```python
from build123d import *

# Parameters (mm, degrees)
SKETCH1_R           = 5.1
BOSS_EXTRUDE1_DEPTH = 5
CUT_EXTRUDE1_START  = -2.3
SKETCH2_R           = 7.5
CUT_EXTRUDE1_DEPTH  = 33.942020373
BOSS_EXTRUDE2_DEPTH = 12
SKETCH4_R           = 5
SKETCH4_R_2         = 1.75
SKETCH4_R_3         = 2.5
CUT_EXTRUDE2_DEPTH  = 37.455291152
FILLET1_R           = 1
SKETCH5_W           = 20
SKETCH5_H           = 6.532082626
CUT_EXTRUDE3_DEPTH  = 37.672994655
FILLET2_R           = 2
FILLET3_R           = 6


with BuildPart() as part:
    # Sketch1 → Boss-Extrude1 (new body)
    with BuildSketch(Plane.XY):
        with BuildLine():
            Line((-27, -16), (27, -16))
            ThreePointArc((27, -16), (29.828427125, -14.828427125), (31, -12))
            Line((31, -12), (31, 12))
            ThreePointArc((31, 12), (29.828427125, 14.828427125), (27, 16))
            Line((27, 16), (-27, 16))
            ThreePointArc((-27, 16), (-29.828427125, 14.828427125), (-31, 12))
            Line((-31, 12), (-31, -12))
            ThreePointArc((-31, -12), (-29.828427125, -14.828427125), (-27, -16))
        make_face()
        with Locations((-20, 9)):
            Circle(SKETCH1_R, mode=Mode.SUBTRACT)
        with Locations((20, -9)):
            Circle(SKETCH1_R, mode=Mode.SUBTRACT)
        with Locations((-20, -9)):
            Circle(SKETCH1_R, mode=Mode.SUBTRACT)
        with Locations((20, 9)):
            Circle(SKETCH1_R, mode=Mode.SUBTRACT)
    extrude(amount=BOSS_EXTRUDE1_DEPTH)

    # Sketch2 → Cut-Extrude1 (cut, through all)
    with BuildSketch(Plane(origin=(0, 0, 0), x_dir=(-1, 0, 0), z_dir=(0, 0, -1)).offset(CUT_EXTRUDE1_START)):
        with Locations((20, 9)):
            Circle(SKETCH2_R)
        with Locations((-20, 9)):
            Circle(SKETCH2_R)
        with Locations((-20, -9)):
            Circle(SKETCH2_R)
        with Locations((20, -9)):
            Circle(SKETCH2_R)
    extrude(amount=-CUT_EXTRUDE1_DEPTH, mode=Mode.SUBTRACT)

    # Sketch3 → Boss-Extrude2 (add, symmetric)
    with BuildSketch(Plane(origin=(0, 0, 0), x_dir=(0, 0, -1), z_dir=(1, 0, 0))):
        Polygon((-5, 16), (-9.770224884, -8.540679586), (-5, -9.467917374), align=None)
        Polygon((0, 16), (-5, 16), (-4.427573014, 18.94488155), (0, 18.94488155), align=None)
    extrude(amount=BOSS_EXTRUDE2_DEPTH, both=True)

    # Sketch4 → Cut-Extrude2 (cut, through all)
    with BuildSketch(Plane(origin=(0, 1.519045647, 7.814812384), x_dir=(1, 0, 0), z_dir=(0, 0.19080899537654522, 0.981627183447664))):
        with Locations(Location((0, 4, 0), (0, 0, 270))):
            Circle(SKETCH4_R)
        with Locations(Location((0, 13, 0), (0, 0, 270))):
            Circle(SKETCH4_R_2)
        with Locations(Location((8, 4, 0), (0, 0, 270))):
            Circle(SKETCH4_R_2)
        with Locations(Location((0, -5, 0), (0, 0, 270))):
            Circle(SKETCH4_R_2)
        with Locations(Location((-8, 4, 0), (0, 0, 270))):
            Circle(SKETCH4_R_2)
        with Locations(Location((-6.686187475, -2.686187475, 0), (0, 0, 270))):
            Circle(SKETCH4_R_3)
        with Locations(Location((6.686187475, -2.686187475, 0), (0, 0, 90))):
            Circle(SKETCH4_R_3)
        with Locations(Location((6.686187475, 10.686187475, 0), (0, 0, 270))):
            Circle(SKETCH4_R_3)
        with Locations(Location((-6.686187475, 10.686187475, 0), (0, 0, 90))):
            Circle(SKETCH4_R_3)
    extrude(amount=-CUT_EXTRUDE2_DEPTH, mode=Mode.SUBTRACT)

    # Fillet1
    # the kernel refuses this fillet: 1 mm, written as the material it adds along each edge
    with BuildSketch(Plane(origin=(12, 16, 0), x_dir=(1, 0, 0), z_dir=(0, 0, 1))) as fillet1_piece_1_section:
        with BuildLine():
            CenterArc((FILLET1_R, FILLET1_R), FILLET1_R, 180, 90)
            Line((0, FILLET1_R), (0, 0))
            Line((0, 0), (FILLET1_R, 0))
        make_face()
    fillet1_piece_1 = extrude(amount=5, mode=Mode.PRIVATE)
    fillet1_piece_1 = split(fillet1_piece_1, bisect_by=Plane(origin=(12.227463764, 16.688764384, 4.866117766), z_dir=(0, -0.19080899537654517, -0.981627183447664)), keep=Keep.TOP, mode=Mode.PRIVATE)
    add(fillet1_piece_1)
    with BuildSketch(Plane(origin=(-12, 16, 0), x_dir=(-1, 0, 0), z_dir=(0, 0, 1))) as fillet1_piece_2_section:
        with BuildLine():
            CenterArc((FILLET1_R, -FILLET1_R), FILLET1_R, 90, 90)
            Line((0, -FILLET1_R), (0, 0))
            Line((0, 0), (FILLET1_R, 0))
        make_face()
    fillet1_piece_2 = extrude(amount=5, mode=Mode.PRIVATE)
    fillet1_piece_2 = split(fillet1_piece_2, bisect_by=Plane(origin=(-12.227463764, 16.688764384, 4.866117766), z_dir=(0, -0.19080899537654517, -0.981627183447664)), keep=Keep.TOP, mode=Mode.PRIVATE)
    add(fillet1_piece_2)
    # the kernel refuses this fillet: 1 mm, written as the material it takes off along each edge
    with BuildSketch(Plane(origin=(12, 18.94488155, 6.927573014), x_dir=(0, -1, 0), z_dir=(0, 0, -1))) as fillet1_2_piece_1:
        with BuildLine():
            CenterArc((FILLET1_R, FILLET1_R), FILLET1_R, 180, 90)
            Line((0, FILLET1_R), (0, 0))
            Line((0, 0), (FILLET1_R, 0))
        make_face()
    extrude(amount=9.427573014, mode=Mode.SUBTRACT)
    with BuildSketch(Plane(origin=(-12, 18.94488155, 6.927573014), x_dir=(0, -1, 0), z_dir=(0, 0, -1))) as fillet1_2_piece_2:
        with BuildLine():
            CenterArc((FILLET1_R, -FILLET1_R), FILLET1_R, 90, 90)
            Line((0, -FILLET1_R), (0, 0))
            Line((0, 0), (FILLET1_R, 0))
        make_face()
    extrude(amount=9.427573014, mode=Mode.SUBTRACT)

    # Sketch5 → Cut-Extrude3 (cut, through all)
    with BuildSketch(Plane.XY.offset(5)):
        with Locations((0, -12.733958687)):
            Rectangle(SKETCH5_W, SKETCH5_H)
    extrude(amount=-CUT_EXTRUDE3_DEPTH, mode=Mode.SUBTRACT)

    # Fillet2
    fillet2_edges = [part.edges().sort_by_distance(p)[0] for p in [
        (-10, -16, 2.5),
        (-10, -9.467917374, 2.5),
        (10, -9.467917374, 2.5),
        (10, -16, 2.5),
    ]]
    fillet(fillet2_edges, radius=FILLET2_R)

    # Fillet3
    # the kernel refuses this fillet: 6 mm, written as the material it takes off along each edge
    with BuildSketch(Plane(origin=(-12, -5.678544656, 24.494632636), x_dir=(1, 0, 0), z_dir=(0, -0.19080899537654505, -0.981627183447664))) as fillet3_piece_1_section:
        with BuildLine():
            CenterArc((FILLET3_R, -FILLET3_R), FILLET3_R, 90, 90)
            Line((0, -FILLET3_R), (0, 0))
            Line((0, 0), (FILLET3_R, 0))
        make_face()
    fillet3_piece_1 = extrude(amount=34.859507728, mode=Mode.PRIVATE)
    fillet3_piece_1 = split(fillet3_piece_1, bisect_by=Plane(origin=(-10.628321285, -7.717365946, 5), z_dir=(0, 0, 1)), keep=Keep.TOP, mode=Mode.PRIVATE)
    add(fillet3_piece_1, mode=Mode.SUBTRACT)
    with BuildSketch(Plane(origin=(12, -5.678544656, 24.494632636), x_dir=(-1, 0, 0), z_dir=(0, -0.19080899537654505, -0.981627183447664))) as fillet3_piece_2_section:
        with BuildLine():
            CenterArc((FILLET3_R, FILLET3_R), FILLET3_R, 180, 90)
            Line((0, FILLET3_R), (0, 0))
            Line((0, 0), (FILLET3_R, 0))
        make_face()
    fillet3_piece_2 = extrude(amount=34.859507728, mode=Mode.PRIVATE)
    fillet3_piece_2 = split(fillet3_piece_2, bisect_by=Plane(origin=(10.628321285, -7.717365946, 5), z_dir=(0, 0, 1)), keep=Keep.TOP, mode=Mode.PRIVATE)
    add(fillet3_piece_2, mode=Mode.SUBTRACT)


solid = part.part
```
Check sheet for the modelled part. Datum: model origin and axes. Units: mm. A direction names the side the tool comes from. Coordinates: 2 decimals unless noted, no trailing zeros. Order: outer loops, then holes, each group sorted by start corner. A loop starts at its lowest first (then second) coordinate and runs counter-clockwise, first axis right, second up. Notation, with made-up numbers: M -37,64.5 L -27,64.5 A21 cw -27,97.5 Z; hole C 81,-34.5 d10. An arc over 180 degrees is marked long. Write each question's results on one line, items separated by ' | '. Start each with the question number.
1. Cross-section at B-B on y = -10.5. Record the cut outline in (x, z), and give its area (3 significant figures).
2. Material ranges on probe 1 along Y at (x, z) = (20, 2.25); probe 2 along X at (y, z) = (-9, 1.55); probe 3 along X at (y, z) = (-8.5, 3.5), recorded low to high.
3. Mould release check, pull along X, two halves, no side actions. Record for faces 5 (the face through (29.859, 14.797, 2.465)), 6 (the face through (22, -1, 5)), 7 (the face through (0, -9.468, 3)): +X half, -X half, draft (parallel to the pull), parting line (faces both ways), or undercut.
4. Cross-section at D-D on x = -23.5. Record the cut outline in (y, z).
5. Cross-section at C-C on z = 1.5. State how many separate pieces and enclosed holes the cut face has, and give its area (3 significant figures).
6. Go/stop test with flat-tipped pins: P1, Ø6, axis at x = 19, y = -8, coming from the -Z side; P2, Ø11.5, axis at x = -19.5, y = -10, coming from the +Z side; P3, Ø2, axis at y = 14, z = 4, coming from the +X side; P4, Ø1.5, axis at x = -16.5, z = 3.5, coming from the +Y side. Record where each tip stops, or that it passes through.
7. Access from +Z, -Z, +X, -X, +Y, -Y to the whole of each face (thin tool, end or side, straight path). Record for faces 1 (the face through (-31, 0, 2)), 2 (the face through (-19.709, 1.506, 3.631)), 3 (the face through (20, 16, 2)), 4 (the face through (9.4, -10.04, 2.46)).
8. Cross-section at A-A on x = 20. Record the cut outline in (y, z), and give its area (3 significant figures).
Checks:
1) outline: M -31,0 L -24.87,0 L -24.87,2.3 L -27.35,2.3 L -27.35,5 L -31,5 Z; M -15.13,0 L -9.75,0 L -9.75,5 L -12.65,5 L -12.65,2.3 L -15.13,2.3 Z; M 9.75,0 L 15.13,0 L 15.13,2.3 L 12.65,2.3 L 12.65,5 L 9.75,5 Z; M 24.87,0 L 31,0 L 31,5 L 27.35,5 L 27.35,2.3 L 24.87,2.3 Z | area: 88.3 mm²
2) probe 1: y = -16 to -14.1, -3.9 to 3.9, 14.1 to 16 | probe 2: x = -31 to -25.1, -14.9 to 14.9, 25.1 to 31 | probe 3: x = -31 to -27.48, -12.52 to 12.52, 27.48 to 31
3) face 5: +X half | face 6: draft | face 7: undercut
4) outline: M -16,0 L -12.71,0 L -12.71,2.3 L -15.63,2.3 L -15.63,5 L -16,5 Z; M -5.29,0 L 5.29,0 L 5.29,2.3 L 2.37,2.3 L 2.37,5 L -2.37,5 L -2.37,2.3 L -5.29,2.3 Z; M 12.71,0 L 16,0 L 16,5 L 15.63,5 L 15.63,2.3 L 12.71,2.3 Z
5) separate pieces: 1 | enclosed holes: 13 | area: 1,380 mm²
6) P1: passes through | P2: stops at z = 2.3 | P3: stops at x = 30.87 | P4: stops at y = 16
7) face 1: +Z, -Z, -X, +Y, -Y | face 2: +Z | face 3: +Z, -Z, +X, +Y | face 4: +Z, -Z, -Y
8) outline: M -16,0 L -14.1,0 L -14.1,2.3 L -16,2.3 Z; M -3.9,0 L 3.9,0 L 3.9,2.3 L 1.5,2.3 L 1.5,5 L -1.5,5 L -1.5,2.3 L -3.9,2.3 Z; M 14.1,0 L 16,0 L 16,2.3 L 14.1,2.3 Z | area: 34.8 mm²
